Input: part model. Units: mm. Frame: model coordinates. A direction names the side the tool comes from. Round coordinates to 2 decimals unless told otherwise and drop trailing zeros. Order: outer loops, then holes, each group sorted by start corner. A loop starts at its lowest first (then second) coordinate and runs counter-clockwise, first axis right, second up. Notation, with made-up numbers: (58.5, 69.5) -> (68.5, 69.5) arc R25 cw to (68.5, 98.5) -> close; hole circle Ø11 at (-19, 49). An arc over 180 degrees is marked (long way). Use a Markdown table: item, result.
from build123d import *

# Parameters (mm, degrees)
F1_DEPTH = 5


with BuildPart() as f1:
    # F0 (on Front) → F1 (new body, symmetric)
    with BuildSketch(Plane.XZ):
        with BuildLine():
            Line((-4.3, 37.6), (-6, 35.776973193))
            Line((-6, 35.776973193), (-21.085353054, -8.0015684709))
            ThreePointArc((-21.085353054, -8.0015684709), (-21.8150214993, -8.9783637404), (-22.9762413446, -9.35))
            Line((-22.9762413446, -9.35), (-58.05, -9.35))
            ThreePointArc((-58.05, -9.35), (-59.4642135624, -8.7642135624), (-60.05, -7.35))
            Line((-60.05, -7.35), (-60.05, -4.85))
            ThreePointArc((-60.05, -4.85), (-60.6357864376, -3.4357864376), (-62.05, -2.85))
            Line((-62.05, -2.85), (-64.55, -2.85))
            ThreePointArc((-64.55, -2.85), (-65.9642135624, -3.4357864376), (-66.55, -4.85))
            Line((-66.55, -4.85), (-66.55, -13.85))
            ThreePointArc((-66.55, -13.85), (-65.9642135624, -15.2642135624), (-64.55, -15.85))
            Line((-64.55, -15.85), (-22.5095066627, -15.85))
            ThreePointArc((-22.5095066627, -15.85), (-21.6444060516, -16.0467803981), (-20.9495402831, -16.5983990675))
            Line((-20.9495402831, -16.5983990675), (-4.3, -37.35))
            Line((-4.3, -37.35), (-4.3, -38.35))
            ThreePointArc((-4.3, -38.35), (-4.0071067812, -39.0571067812), (-3.3, -39.35))
            Line((-3.3, -39.35), (7.45, -39.35))
            Line((7.45, -39.35), (7.45, -42.55))
            Line((7.45, -42.55), (6.7, -42.55))
            Line((6.7, -42.55), (6.7, -44.25))
            ThreePointArc((6.7, -44.25), (6.8464466094, -44.6035533906), (7.2, -44.75))
            Line((7.2, -44.75), (9.7, -44.75))
            ThreePointArc((9.7, -44.75), (10.0535533906, -44.6035533906), (10.2, -44.25))
            Line((10.2, -44.25), (10.2, -36.15))
            ThreePointArc((10.2, -36.15), (9.9071067812, -35.4428932188), (9.2, -35.15))
            Line((9.2, -35.15), (1, -35.15))
            ThreePointArc((1, -35.15), (0.2928932188, -34.8571067812), (0, -34.15))
            Line((0, -34.15), (0, 34.15))
            ThreePointArc((0, 34.15), (0.5857864376, 35.5642135624), (2, 36.15))
            Line((2, 36.15), (8.4, 36.15))
            Line((8.4, 36.15), (8.4, 32.15))
            ThreePointArc((8.4, 32.15), (8.6928932188, 31.4428932188), (9.4, 31.15))
            Line((9.4, 31.15), (9.7, 31.15))
            ThreePointArc((9.7, 31.15), (10.4071067812, 31.4428932188), (10.7, 32.15))
            Line((10.7, 32.15), (10.7, 39.6))
            Line((10.7, 39.6), (12.0584372697, 41.1197607825))
            ThreePointArc((12.0584372697, 41.1197607825), (12.5542284753, 42.2243517405), (12.3218441058, 43.4125973417))
            Line((12.3218441058, 43.4125973417), (9.6272657122, 48.3374442137))
            ThreePointArc((9.6272657122, 48.3374442137), (8.7116734449, 50.6601925206), (8.4, 53.1373539124))
            Line((8.4, 53.1373539124), (8.4, 56.1))
            ThreePointArc((8.4, 56.1), (8.1071067812, 56.8071067812), (7.4, 57.1))
            Line((7.4, 57.1), (7.1, 57.1))
            ThreePointArc((7.1, 57.1), (6.3928932188, 56.8071067812), (6.1, 56.1))
            Line((6.1, 56.1), (6.1, 53.1373539124))
            ThreePointArc((6.1, 53.1373539124), (6.4116734449, 50.6601925206), (7.3272657122, 48.3374442137))
            Line((7.3272657122, 48.3374442137), (10.0218441058, 43.4125973417))
            ThreePointArc((10.0218441058, 43.4125973417), (10.2542284753, 42.2243517405), (9.7584372697, 41.1197607825))
            Line((9.7584372697, 41.1197607825), (8.4, 39.6))
            Line((8.4, 39.6), (-3.3, 39.6))
            ThreePointArc((-3.3, 39.6), (-4.0071067812, 39.3071067812), (-4.3, 38.6))
            Line((-4.3, 38.6), (-4.3, 37.6))
        make_face()
        with BuildLine():
            Line((-6, 12.8393314671), (-6, -23.4222970219))
            ThreePointArc((-6, -23.4222970219), (-6.334162425, -23.8939938512), (-6.8899915949, -23.7351972551))
            Line((-6.8899915949, -23.7351972551), (-15.8036005744, -12.6254817154))
            Line((-15.8036005744, -12.6254817154), (-6.9727220727, 13.0022235849))
            ThreePointArc((-6.9727220727, 13.0022235849), (-6.417419846, 13.3324648347), (-6, 12.8393314671))
        make_face(mode=Mode.SUBTRACT)
    extrude(amount=F1_DEPTH, both=True)


solid = f1.part
1) Cut plane C-C on x = -27.5. Return loops of the section in (y, z), and give its area (3 significant figures).
Results found:
| item | result |
|---|---|
| outline | (-5, -15.85) -> (5, -15.85) -> (5, -9.35) -> (-5, -9.35) -> close |
| area | 65.0 mm² |
2) Pin query (flat end, axial travel): pin 1 Ø1.4 at (y, z) = (-2, -44) entering from -X; pin 2 Ø3 at (y, z) = (1.5, 34) entering from -X; pin 3 Ø4 at (x, y) = (-5, 0) entering from +Z. Return the tip coordinate at first contact, or that it passes through.
Results found:
| item | result |
|---|---|
| pin 1 | stops at x = 6.7 |
| pin 2 | stops at x = -7.13 |
| pin 3 | stops at z = 39.6 |
3) Cut plane B-B on x = -13.5. Return loops of the section in (y, z), and give its area (3 significant figures).
Results found:
| item | result |
|---|---|
| outline | (-5, -25.88) -> (5, -25.88) -> (5, -15.5) -> (-5, -15.5) -> close; (-5, -5.94) -> (5, -5.94) -> (5, 14.01) -> (-5, 14.01) -> close |
| area | 303 mm² |
4) Cut plane A-A on z = 11. Return loops of the section in (x, y), and give its area (3 significant figures).
Results found:
| item | result |
|---|---|
| outline | (-14.54, -5) -> (-7.66, -5) -> (-7.66, 5) -> (-14.54, 5) -> close; (-6, -5) -> (0, -5) -> (0, 5) -> (-6, 5) -> close |
| area | 129 mm² |
5) Pull-direction query (Z, two-part tool) for faces 1 (the cylindrical face through (10.256, -0.07, 42.241)), 2 (the cylindrical face through (12.552, -0.07, 42.207)), 3 (the cylindrical face through (0.57, -0.07, 35.55)), 4 (the flat face through (-66.55, 0, -9)); classes: +Z half, -Z half, draft (parallel to the pull), parting line (faces both ways), or undercut.
Results found:
| item | result |
|---|---|
| face 1 | undercut |
| face 2 | parting line |
| face 3 | undercut |
| face 4 | draft |
6) Set-up query: faces 5 (the flat face through (5, 0, 36.15)), 6 (the flat face through (-63, 0, -2.85)), 7 (the flat face through (10.7, 0, 36)), 8 (the flat face through (3, 0, 39.6)), 9 (the cylindrical face through (-60.62, -0.07, -3.45)). Return all of +Z, -Z, +X, -X, +Y, -Y with unobstructed straight access to the full face (end or side cutting, diameter ignored); none if empty.
Results found:
| item | result |
|---|---|
| face 5 | +Y, -Y |
| face 6 | +Z, -X, +Y, -Y |
| face 7 | -Z, +X, +Y, -Y |
| face 8 | -X, +Y, -Y |
| face 9 | +Z, +Y, -Y |
7) Line query: L1, parallel to X at y = 0.25, z = -7.5; L2, parallel to Z at x = -37.5, y = 2.5; L3, parallel to Z at x = 6, y = -1.75. Output: solid intervals per line, ascending. Write a range as [from, to].
Results found:
| item | result |
|---|---|
| L1 | x = [-66.55, -60.04], [-20.91, -14.04], [-6, 0] |
| L2 | z = [-15.85, -9.35] |
| L3 | z = [-39.35, -35.15], [36.15, 39.6] |
8) Cut plane D-D on z = 26. Return loops of the section in (x, y).
Results found:
| item | result |
|---|---|
| outline | (-9.37, -5) -> (0, -5) -> (0, 5) -> (-9.37, 5) -> close |
